from build123d import *

# Parameters (mm, degrees)
BOSS_EXTRUDE1_DEPTH = 10
SKETCH2_R           = 0.7
CUT_EXTRUDE1_DEPTH  = 10
CIRPATTERN3_COUNT   = 20
FILLET1_R           = 0.2
CUT_EXTRUDE2_REACH  = 12
SKETCH3_R           = 3.5
SKETCH4_W           = 0.6
SKETCH4_H           = 10.414964042
BOSS_EXTRUDE2_DEPTH = 10


with BuildPart() as part:
    # Sketch1 → Boss-Extrude1 (new body)
    with BuildSketch(Plane(origin=(0, 0, 0), x_dir=(1, 0, 0), z_dir=(0, 1, 0))):
        Polygon((4.951468525, -3.59745246), (5.820800352, -1.891292682), (6.120351685, 0), (5.820800352, 1.891292682), (4.951468525, 3.59745246), (3.59745246, 4.951468525), (1.891292682, 5.820800352), (0, 6.120351685), (-1.891292682, 5.820800352), (-3.59745246, 4.951468525), (-4.951468525, 3.59745246), (-5.820800352, 1.891292682), (-6.120351685, 0), (-5.820800352, -1.891292682), (-4.951468525, -3.59745246), (-3.59745246, -4.951468525), (-1.891292682, -5.820800352), (0, -6.120351685), (1.891292682, -5.820800352), (3.59745246, -4.951468525), align=None)
    extrude(amount=BOSS_EXTRUDE1_DEPTH)

    # Sketch2 → Cut-Extrude1 (cut)
    with BuildSketch(Plane(origin=(0, 10, 0), x_dir=(1, 0, 0), z_dir=(0, 1, 0))):
        with Locations((5.855, 0)):
            Circle(SKETCH2_R)
    cut_extrude1 = extrude(amount=-CUT_EXTRUDE1_DEPTH, mode=Mode.SUBTRACT)

    # CirPattern3: Cut-Extrude1 ×20 about axis
    cirpattern3_axis = Axis((-0.052482021, 0, 0), (0, 1, 0))
    for i in range(1, CIRPATTERN3_COUNT):
        add(cut_extrude1.rotate(cirpattern3_axis, i * 360 / CIRPATTERN3_COUNT), mode=Mode.SUBTRACT)

    # Fillet1
    fillet1_edges = [part.edges().sort_by_distance(p)[0] for p in [
        (4.057798917, 5, -4.491122068),
        (2.93831654, 5, -5.287315051),
        (5.251367741, 5, -3.008867108),
        (4.438640047, 5, -4.110280937),
        (2.467098423, 5, -5.527412673),
        (1.150354408, 5, -5.938153446),
        (0.638542887, 5, -6.019216428),
        (-0.746045616, 5, -6.002189668),
        (-1.247642454, 5, -5.922744534),
        (-2.563808053, 5, -5.478136656),
        (-3.008267267, 5, -5.251673375),
        (-4.126835407, 5, -4.422085577),
        (-4.474567598, 5, -4.074353387),
        (-5.286407893, 5, -2.940096937),
        (-5.507494847, 5, -2.506189359),
        (-5.933957193, 5, -1.176848512),
        (-6.009763498, 5, -0.698226334),
        (-6.009763498, 5, 0.698226334),
        (-5.933957193, 5, 1.176848512),
        (-5.507494847, 5, 2.506189359),
        (-5.286407893, 5, 2.940096937),
        (-4.474567598, 5, 4.074353387),
        (-4.126835407, 5, 4.422085577),
        (-3.008267267, 5, 5.251673375),
        (-2.563808053, 5, 5.478136656),
        (-1.247642454, 5, 5.922744534),
        (-0.746045616, 5, 6.002189668),
        (0.638542887, 5, 6.019216428),
        (1.150354408, 5, 5.938153446),
        (2.467098423, 5, 5.527412673),
        (2.93831654, 5, 5.287315051),
        (4.057798917, 5, 4.491122068),
        (5.251367741, 5, 3.008867108),
        (4.438640047, 5, 4.110280937),
        (5.499267273, 5, 2.522336881),
        (5.926264611, 5, 1.225417561),
        (5.926264611, 5, -1.225417561),
        (5.499267273, 5, -2.522336881),
        (6.012318774, 5, 0.682092958),
        (6.012318774, 5, -0.682092958),
    ]]
    fillet(fillet1_edges, radius=FILLET1_R)

    # Sketch3 → Cut-Extrude2 (cut, up to next)
    with BuildSketch(Plane(origin=(0, 10, 0), x_dir=(1, 0, 0), z_dir=(0, 1, 0)), mode=Mode.PRIVATE) as cut_extrude2_sk1:
        with Locations(Location((0, 0, 0), (0, 0, 270))):  # turned: the seam where the file's is
            Circle(SKETCH3_R)
    cut_extrude2_tool1 = extrude(cut_extrude2_sk1.sketch, amount=-CUT_EXTRUDE2_REACH, mode=Mode.PRIVATE) & part.part
    add(cut_extrude2_tool1.solids().sort_by_distance((0, 10, 0))[0], mode=Mode.SUBTRACT)

    # Sketch4 → Boss-Extrude2 (add)
    with BuildSketch(Plane.XZ):
        Rectangle(SKETCH4_W, SKETCH4_H)
    extrude(amount=-BOSS_EXTRUDE2_DEPTH)


solid = part.part
The listing builds one solid part. Answer for the finished solid, in the listing's coordinates (mm). A direction names the side the tool comes from. Give positions to 0.01 mm unless a question says otherwise; leave off trailing zeros. Write each loop counter-clockwise with the first axis right and the second up, starting at its lowest first coordinate (ties: lowest second). Pieces come first, ordered by that corner, then holes.
1) Section C-C (x = -3.25) is taken. Write down the section's boundary in (y, z).
2) Section B-B (x = 1.25) is taken. Write down the section's boundary in (y, z), and give its area (3 significant figures).
3) Section D-D (z = 2) is taken. Write down the section's boundary in (x, y), and give its area (3 significant figures).
4) Find the intervals of material crossed by L1, parallel to X at y = 4.5, z = 0 (3 decimals); L2, parallel to X at y = 0.5, z = -4.25; L3, parallel to X at y = 8.5, z = 4.75, in increasing order.
5) Section A-A (z = 0) is taken. Write down the section's boundary in (x, y) (3 decimals), and give its area (3 significant figures).
6) Given P1, Ø5, axis at x = 3, z = 2, coming from the -Y side; P2, Ø3, axis at x = 3, y = 8.5, coming from the +Z side; P3, Ø4, axis at y = 5, z = -3, coming from the -X side; P4, Ø1, axis at x = -1.5, y = 6, coming from the +Z side, each flat-ended and moving along its own axis, determine where each tip first touches the part or whether it passes through.
7) For a pull along Z with two mould halves and no side action, classify faces 3 (the face through (-0.032, 5.07, 5.208)), 4 (the face through (4.17, 5.07, 3.05)), 5 (the face through (0, 0, 0)) as pulls with the +Z half, pulls with the -Z half, needs draft (parallel to the pull), parting line crosses it, or undercut.
8) A tool of negligible diameter and unlimited length cuts with its end or side. For faces 1 (the face through (5.155, 5.07, -0.015)), 2 (the face through (-3.5, 5.1, -0.1)), from which of +Z, -Z, +X, -X, +Y, -Y can it reach the whole face along a straight path? Write none if from no direction.
Response:
1. outline: (0, -4.14) - (10, -4.14) - (10, -1.3) - (0, -1.3) - close; (0, 1.3) - (10, 1.3) - (10, 4.14) - (0, 4.14) - close
2. outline: (0, -5.15) - (10, -5.15) - (10, -3.27) - (0, -3.27) - close; (0, 3.27) - (10, 3.27) - (10, 5.15) - (0, 5.15) - close
2. area: 37.7 mm2
3. outline: (-4.99, 0) - (-2.87, 0) - (-2.87, 10) - (-4.99, 10) - close; (-0.3, 0) - (0.3, 0) - (0.3, 10) - (-0.3, 10) - close; (2.87, 0) - (4.89, 0) - (4.89, 10) - (2.87, 10) - close
3. area: 47.4 mm2
4. L1: x = -5.26 to -3.5, -0.3 to 0.3, 3.5 to 5.155
4. L2: x = -4.3 to -3.98, -3.07 to 2.96, 3.88 to 4.29
4. L3: x = -2.83 to 2.72
5. outline: (-5.26, 0) - (-3.5, 0) - (-3.5, 10) - (-5.26, 10) - close; (-0.3, 0) - (0.3, 0) - (0.3, 10) - (-0.3, 10) - close; (3.5, 0) - (5.155, 0) - (5.155, 10) - (3.5, 10) - close
5. area: 40.1 mm2
6. P1: stops at y = 0
6. P2: stops at z = 5.44
6. P3: stops at x = -5.96
6. P4: stops at z = 5.96
7. face 3: pulls with the +Z half
7. face 4: undercut
7. face 5: needs draft
8. face 1: +X, +Y, -Y
8. face 2: +Y, -Y
